For this review, take the finished solid that the model builds, in its own axes (mm). Coordinates: 2 decimals unless noted, no trailing zeros. Write each loop counter-clockwise with the first axis right and the second up, starting at its lowest first coordinate (ties: lowest second). Pieces come first, ordered by that corner, then holes.
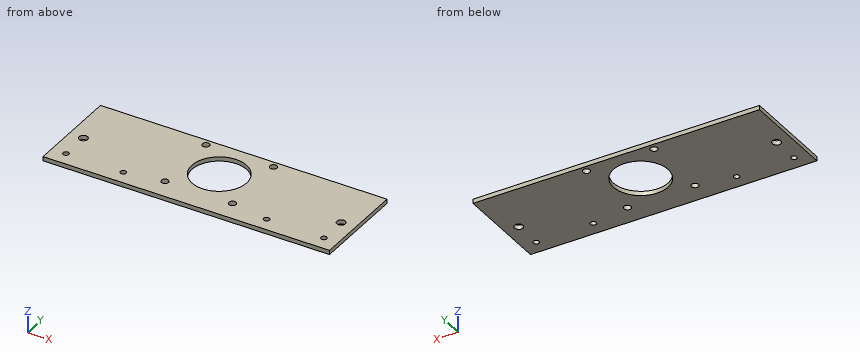
```python
from build123d import *

# Parameters (mm, degrees)
SKIZZE1_W                       = 200
SKIZZE1_H                       = 66.2
AUFSATZ_LINEAR_AUSTRAGEN1_DEPTH = 3
SKIZZE2_R                       = 19.0625
SCHNITT_LINEAR_AUSTRAGEN1_DEPTH = 24
SKIZZE3_R                       = 2
SCHNITT_LINEAR_AUSTRAGEN2_DEPTH = 10
SKIZZE4_R                       = 3
SCHNITT_LINEAR_AUSTRAGEN3_DEPTH = 10
SKIZZE5_R                       = 2.5
SCHNITT_LINEAR_AUSTRAGEN4_DEPTH = 10


with BuildPart() as part:
    # Skizze1 → Aufsatz-Linear austragen1 (new body)
    with BuildSketch(Plane.XY):
        with Locations((100, 33.1)):
            Rectangle(SKIZZE1_W, SKIZZE1_H)
    extrude(amount=AUFSATZ_LINEAR_AUSTRAGEN1_DEPTH)

    # Skizze2 → Schnitt-Linear austragen1 (cut)
    with BuildSketch(Plane.XY.offset(3)):
        with Locations((100, 38)):
            Circle(SKIZZE2_R)
    extrude(amount=-SCHNITT_LINEAR_AUSTRAGEN1_DEPTH, mode=Mode.SUBTRACT)

    # Skizze3 → Schnitt-Linear austragen2 (cut)
    with BuildSketch(Plane(origin=(0, 0, 0), x_dir=(-1, 0, 0), z_dir=(0, 0, -1))):
        with Locations((-190, 10)):
            Circle(SKIZZE3_R)
        with Locations((-150, 10)):
            Circle(SKIZZE3_R)
        with Locations((-50, 10)):
            Circle(SKIZZE3_R)
        with Locations((-10, 10)):
            Circle(SKIZZE3_R)
    extrude(amount=-SCHNITT_LINEAR_AUSTRAGEN2_DEPTH, mode=Mode.SUBTRACT)

    # Skizze4 → Schnitt-Linear austragen3 (cut)
    with BuildSketch(Plane(origin=(0, 0, 0), x_dir=(-1, 0, 0), z_dir=(0, 0, -1))):
        with Locations((-190, 30)):
            Circle(SKIZZE4_R)
        with Locations((-10, 30)):
            Circle(SKIZZE4_R)
    extrude(amount=-SCHNITT_LINEAR_AUSTRAGEN3_DEPTH, mode=Mode.SUBTRACT)

    # Skizze5 → Schnitt-Linear austragen4 (cut)
    with BuildSketch(Plane(origin=(0, 0, 0), x_dir=(-1, 0, 0), z_dir=(0, 0, -1))):
        with Locations((-76.43, 61.57)):
            Circle(SKIZZE5_R)
        with Locations((-123.57, 61.57)):
            Circle(SKIZZE5_R)
        with Locations((-123.57, 14.43)):
            Circle(SKIZZE5_R)
        with Locations((-76.43, 14.43)):
            Circle(SKIZZE5_R)
    extrude(amount=-SCHNITT_LINEAR_AUSTRAGEN4_DEPTH, mode=Mode.SUBTRACT)


solid = part.part
```
Q1. Add section B-B (y = 61.57). State the section outline as (x, z) points, then the cut area to 3 significant figures.
Ans:
outline: (0, 0) - (73.93, 0) - (73.93, 3) - (0, 3) - close; (78.93, 0) - (121.07, 0) - (121.07, 3) - (78.93, 3) - close; (126.07, 0) - (200, 0) - (200, 3) - (126.07, 3) - close
area: 570 mm2
Q2. Add section A-A (x = 100). State the section outline as (y, z) points.
Ans:
outline: (0, 0) - (18.94, 0) - (18.94, 3) - (0, 3) - close; (57.06, 0) - (66.2, 0) - (66.2, 3) - (57.06, 3) - close
Q3. For probe 1 along Y at (x, z) = (76.43, 1.6); probe 2 along Y at (x, z) = (190, 1.25); probe 3 along X at (y, z) = (11.5, 1.6), list the stretches that pass through material, from the lowest coordinate up.
Ans:
probe 1: y = 0 to 11.93, 16.93 to 59.07, 64.07 to 66.2
probe 2: y = 0 to 8, 12 to 27, 33 to 66.2
probe 3: x = 0 to 8.68, 11.32 to 48.68, 51.32 to 148.68, 151.32 to 188.68, 191.32 to 200
Q4. Clearance check with flat-ended pins moving along their axes: pin 1 Ø5 at (x, y) = (10, 10) entering from +Z; pin 2 Ø4.5 at (x, y) = (123.57, 61.57) entering from -Z. State where each tip first meets the part, or that it passes through.
Ans:
pin 1: stops at z = 3
pin 2: passes through
Q5. Add section D-D (z = 0.8). Give the number of separate pieces and of enclosed holes in the cut face, then the cut area to 3 significant figures.
Ans:
separate pieces: 1
enclosed holes: 11
area: 11,900 mm2
Q6. Add section C-C (y = 38). State the section outline as (x, z) points, then the cut area to 3 significant figures.
Ans:
outline: (0, 0) - (80.94, 0) - (80.94, 3) - (0, 3) - close; (119.06, 0) - (200, 0) - (200, 3) - (119.06, 3) - close
area: 486 mm2
